For this review, take the finished solid that the model builds, in its own axes (mm). A direction names the side the tool comes from. Round coordinates to 2 decimals unless told otherwise and drop trailing zeros. Order: outer loops, then holes, each group sorted by start corner. A loop starts at its lowest first (then second) coordinate and runs counter-clockwise, first axis right, second up. Notation, with made-up numbers: (71, -31) - (106, -31) arc R13 ccw to (106, -10) - close; hole circle Ø5 at (44, -0.5). An arc over 180 degrees is marked (long way). One line per item, written item: value.
```python
from build123d import *

# Parameters (mm, degrees)
CROQUIS1_R              = 12.5
SALIENTE_EXTRUIR1_DEPTH = 119
CROQUIS5_R              = 6
CORTAR_EXTRUIR1_DEPTH   = 30


with BuildPart() as part:
    # Croquis1 → Saliente-Extruir1 (new body)
    with BuildSketch(Plane.XY):
        Circle(CROQUIS1_R)
    extrude(amount=SALIENTE_EXTRUIR1_DEPTH)

    # Croquis4 → Revolución1 (revolve)
    with BuildSketch(Plane(origin=(0, 0, 0), x_dir=(0, 0, -1), z_dir=(1, 0, 0)), mode=Mode.PRIVATE) as revoluci_n1_sk:
        with BuildLine():
            Line((-119, 0), (-126.5, 0))
            Line((-126.5, 0), (-126.5, -8.870082917))
            ThreePointArc((-126.5, -8.870082917), (-126.266044443, -9.512870527), (-125.673648178, -9.85489067))
            Line((-125.673648178, -9.85489067), (-124, -10.15))
            Line((-124, -10.15), (-121.5, -10.15))
            Line((-121.5, -10.15), (-121.5, -11.5))
            Line((-121.5, -11.5), (-120.732050808, -11.5))
            Line((-120.732050808, -11.5), (-119, -12.5))
            Line((-119, -12.5), (-119, 0))
        make_face()
    revolve(revoluci_n1_sk.sketch.rotate(Axis((0, 0, 119), (0, 0, 1)), 180), axis=Axis((0, 0, 119), (0, 0, 1)))

    # Croquis5 → Cortar-Extruir1 (cut)
    with BuildSketch(Plane(origin=(0, 0, 0), x_dir=(-1, 0, 0), z_dir=(0, 0, -1))):
        Circle(CROQUIS5_R)
    extrude(amount=-CORTAR_EXTRUIR1_DEPTH, mode=Mode.SUBTRACT)


solid = part.part
```
Item 1: Machinability: for faces 4 (the flat face through (0, 0, 126.5)), 5 (the flat face through (8, -7, 121.5)), 6 (the flat face through (0, 0, 30)), which of the approach directions +Z, -Z, +X, -X, +Y, -Y give a long, thin tool a straight path to every point of the face, cutting with its end or side? Answer none if there is none.
Returned:
face 4: +Z, +X, -X, +Y, -Y
face 5: +Z
face 6: -Z
Item 2: Take a section at D-D (z = 104.5). Write out the cut boundary in (x, y).
Returned:
outline: circle Ø25 at (0, 0)
Item 3: Take a section at A-A (y = 0). Write out the cut boundary in (x, z).
Returned:
outline: (-12.5, 0) - (-6, 0) - (-6, 30) - (6, 30) - (6, 0) - (12.5, 0) - (12.5, 119) - (11.5, 120.73) - (11.5, 121.5) - (10.15, 121.5) - (10.15, 124) - (9.85, 125.67) arc R1 ccw to (8.87, 126.5) - (-8.87, 126.5) arc R1 ccw to (-9.85, 125.67) - (-10.15, 124) - (-10.15, 121.5) - (-11.5, 121.5) - (-11.5, 120.73) - (-12.5, 119) - close
Item 4: For P1, Ø4, axis at y = 8.5, z = 105, coming from the -X side; P2, Ø3, axis at x = 3.5, z = 16, coming from the -Y side; P3, Ø5, axis at x = -9, z = 53.5, coming from the +Y side, all flat-tipped, find the tip position at first contact; note any pin that passes through.
Returned:
P1: x = -10.68
P2: y = -12.34
P3: y = 10.68
Item 5: Wall thickness on line 1 (Y direction, x = 0, z = 16); line 2 (Z direction, x = 4.75, y = 2.75); line 3 (X direction, y = -0.25, z = 102): over which ranges is each line inside the solid? List them lowest first.
Returned:
line 1: -12.5 to -6, 6 to 12.5
line 2: 30 to 126.5
line 3: -12.5 to 12.5
Item 6: Take a section at C-C (z = 8.5). Write out the cut boundary in (x, y), plus the area to 3 significant figures.
Returned:
outline: circle Ø25 at (0, 0); hole circle Ø12 at (0, 0)
area: 378 mm^2
Item 7: The part is to be moulded in two halves that separate along Y. For faces 1 (the cylindrical face through (6, 0, 15)), 2 (the cylindrical face through (6.18, -8.05, 122.73)), 3 (the flat face through (-3, -5.4, 0)), say which applies: +Y half, -Y half, draft (parallel to the pull), parting line (faces both ways), or undercut.
Returned:
face 1: undercut
face 2: parting line
face 3: draft
